```python
from build123d import *

# Parameters (mm, degrees)
SKETCH1_W           = 75
SKETCH1_H           = 75
BOSS_EXTRUDE1_DEPTH = 700
SKETCH2_2_W         = 20
SKETCH2_2_H         = 10
SKETCH2_2_W_2       = 10
SKETCH2_2_H_2       = 20
CUT_EXTRUDE2_DEPTH  = 435
SKETCH2_4_W         = 10
SKETCH2_4_H         = 20
CUT_EXTRUDE3_DEPTH  = 701


with BuildPart() as part:
    # Sketch1 → Boss-Extrude1 (new body)
    with BuildSketch(Plane(origin=(0, 0, 0), x_dir=(1, 0, 0), z_dir=(0, 1, 0))):
        Rectangle(SKETCH1_W, SKETCH1_H)
    extrude(amount=BOSS_EXTRUDE1_DEPTH)

    # Sketch2_2 → Cut-Extrude2 (cut)
    with BuildSketch(Plane(origin=(0, 700, 0), x_dir=(1, 0, 0), z_dir=(0, 1, 0))):
        with Locations((0, -32.5)):
            Rectangle(SKETCH2_2_W, SKETCH2_2_H)
        with Locations((-32.5, 0)):
            Rectangle(SKETCH2_2_W_2, SKETCH2_2_H_2)
    extrude(amount=-CUT_EXTRUDE2_DEPTH, mode=Mode.SUBTRACT)

    # Sketch2_4 → Cut-Extrude3 (cut, through all)
    with BuildSketch(Plane(origin=(0, 700, 0), x_dir=(1, 0, 0), z_dir=(0, 1, 0))):
        with Locations((32.5, 0)):
            Rectangle(SKETCH2_4_W, SKETCH2_4_H)
    extrude(amount=-CUT_EXTRUDE3_DEPTH, mode=Mode.SUBTRACT)


solid = part.part
```
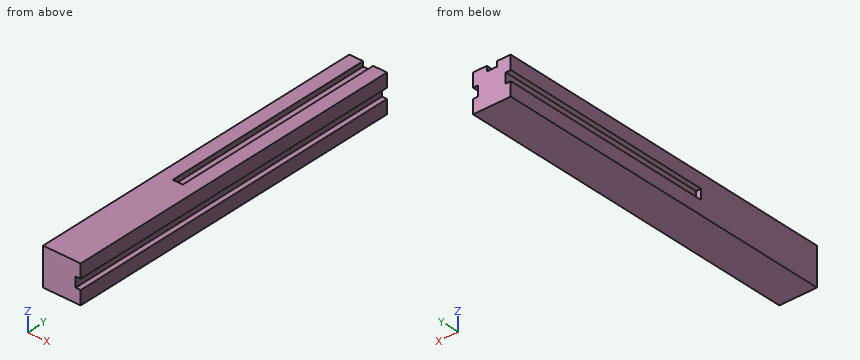
Build history of the part. All positions in model axes, mm. Coordinates: 2 decimals unless noted, no trailing zeros. Order: outer loops, then holes, each group sorted by start corner. A loop starts at its lowest first (then second) coordinate and runs counter-clockwise, first axis right, second up. Notation, with made-up numbers: (67, -18) -> (77, -18) arc R29 cw to (77, 7) -> close; hole circle Ø7 at (35, -10). An arc over 180 degrees is marked (long way). Answer in a Markdown table with one row per item. Add a question column.
Q1. Band-saw the part on B-B, the plane z = 0.5. List the corners of the cut face in (x, y), then the cut area to 4 significant figures.
Q2. Drop flat-ended pins along their axis: pin 1 (6 mm diameter, centred on y = 415.5, z = -3.5, fed in from -X); pin 2 (16 mm diameter, centred on x = 1.5, y = 515.5, fed in from +Z); pin 3 (10 mm diameter, centred on y = 374.5, z = -3, fed in from +X). Give the stop position or say it passes through.
Q3. Wall check: line 1 along X through (y, z) = (517.5, -1.5); line 2 along Z through (x, y) = (-30.5, 414); line 3 along Z through (x, y) = (6, 533.5). Give the ranges that are in metal, low to high. Write a range as [from, to].
Q4. Band-saw the part on A-A, the plane y = 210. List the corners of the cut face in (x, z).
Answers follow:
| question | item | result |
|---|---|---|
| 1 | outline | (-37.5, 0) -> (27.5, 0) -> (27.5, 700) -> (-27.5, 700) -> (-27.5, 265) -> (-37.5, 265) -> close |
| 1 | area | 41,150 mm^2 |
| 2 | pin 1 | x = -27.5 |
| 2 | pin 2 | z = 27.5 |
| 2 | pin 3 | x = 27.5 |
| 3 | line 1 | [-27.5, 27.5] |
| 3 | line 2 | [-37.5, -10], [10, 37.5] |
| 3 | line 3 | [-37.5, 27.5] |
| 4 | outline | (-37.5, -37.5) -> (37.5, -37.5) -> (37.5, -10) -> (27.5, -10) -> (27.5, 10) -> (37.5, 10) -> (37.5, 37.5) -> (-37.5, 37.5) -> close |
